```python
from build123d import *

# Parameters (mm, degrees)
F4_DEPTH = 12


with BuildPart() as f1:
    # F0 (on Top) → F1 (revolve)
    with BuildSketch(Plane.XY):
        Polygon((-30, 10), (0, 10), (0, 18), (-76, 18), (-96, 54), (-100, 54), (-100, 50), (-99.777778, 50), (-82, 18), (-88, 18), (-88, 10), (-60, 10), (-60, 12), (-30, 12), align=None)
    revolve(axis=Axis((-50, 0, 0), (1, 0, 0)))

    # F3 (on offset) → F4 (join)
    with BuildSketch(Plane.XZ.offset(-54)):
        with BuildLine():
            Line((-100, 43), (-100, -43))
            Line((-100, -43), (-20, -43))
            ThreePointArc((-20, -43), (-16.464466, -41.535534), (-15, -38))
            Line((-15, -38), (-15, 38))
            ThreePointArc((-15, 38), (-16.464466, 41.535534), (-20, 43))
            Line((-20, 43), (-100, 43))
        make_face()
    extrude(amount=F4_DEPTH)


solid = f1.part
```
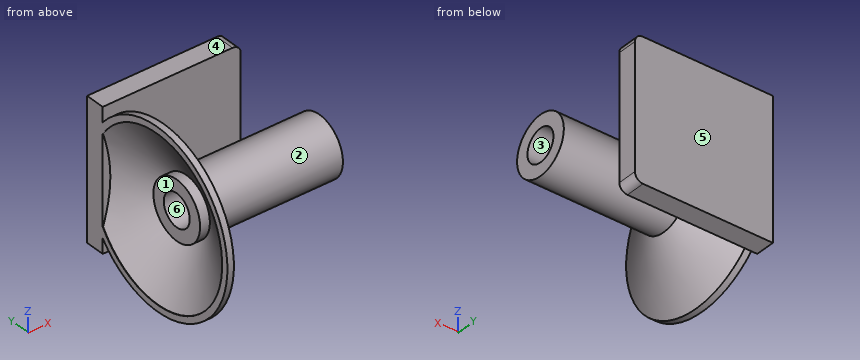
Part model, mm, in its own coordinate system. Face numbers are marked on the shaded views. A direction names the side the tool comes from. Round coordinates to 2 decimals unless told otherwise and drop trailing zeros. Order: outer loops, then holes, each group sorted by start corner. A loop starts at its lowest first (then second) coordinate and runs counter-clockwise, first axis right, second up. Notation, with made-up numbers: M 20.25,-30 L 36.25,-30 A30 cw 36.25,-7 Z; hole C -37.5,-35.5 d8. An arc over 180 degrees is marked long. Answer in a Markdown table with one row per item. Add a question column.
Q1. 3-axis set-ups, long thin cutter, end or side, ignore diameter. For the marked faces 1, 2 and 3: which of +Z, -Z, +X, -X, +Y, -Y reach the whole face in a straight line?
Q2. Cut at A-A on x = -79.5. Give the cut face in (y, z).
Q3. Cut at C-C on x = -68.5. Give the cut face in (y, z).
Q4. Mould opens along Z. For the marked faces 4, 5 and 6 say: +Z half, -Z half, draft (parallel to the pull), parting line (faces both ways), or undercut.
Q5. Wall check: L1, parallel to Z at x = -99.85, y = 0; L2, parallel to Z at x = -10.25, y = 0; L3, parallel to X at y = -12, z = -12. Give the ranges that are in metal, low to high. Write a range as from..to.
Q6. Cut at B-B on y = 0. Give the cut face in (x, z).
Q7. Pin check, flat tips, straight feed: pin 1 (4 mm diameter, centred on y = -35.5, z = 28.5, fed in from +X); pin 2 (1 mm diameter, centred on x = -50.5, z = -22.5, fed in from -Y); pin 3 (18 mm diameter, centred on y = 0, z = 0, fed in from +X) (1 decimal); pin 4 (6 mm diameter, centred on y = 50.5, z = -13.5, fed in from +X). Stop position of each tip, or through.
Established:
| question | item | result |
|---|---|---|
| 1 | face 1 | -X |
| 1 | face 2 | +X |
| 1 | face 3 | +X, -X |
| 2 | outline | C 0,0 d48.6; M 42,-43 L 54,-43 L 54,43 L 42,43 Z; hole C 0,0 d20 |
| 3 | outline | C 0,0 d36; M 42,-43 L 54,-43 L 54,43 L 42,43 Z; hole C 0,0 d20 |
| 4 | face 4 | +Z half |
| 4 | face 5 | draft |
| 4 | face 6 | undercut |
| 5 | L1 | z = -54..-50, 50..54 |
| 5 | L2 | z = -18..-10, 10..18 |
| 5 | L3 | x = -88..0 |
| 6 | outline | M -100,-54 L -96,-54 L -76,-18 L 0,-18 L 0,-10 L -30,-10 L -30,-12 L -60,-12 L -60,-10 L -88,-10 L -88,-18 L -82,-18 L -99.78,-50 L -100,-50 Z; M -100,50 L -99.78,50 L -82,18 L -88,18 L -88,10 L -60,10 L -60,12 L -30,12 L -30,10 L 0,10 L 0,18 L -76,18 L -96,54 L -100,54 Z |
| 7 | pin 1 | stops at x = -90.18 |
| 7 | pin 2 | stops at y = 42 |
| 7 | pin 3 | passes through |
| 7 | pin 4 | stops at x = -15 |
